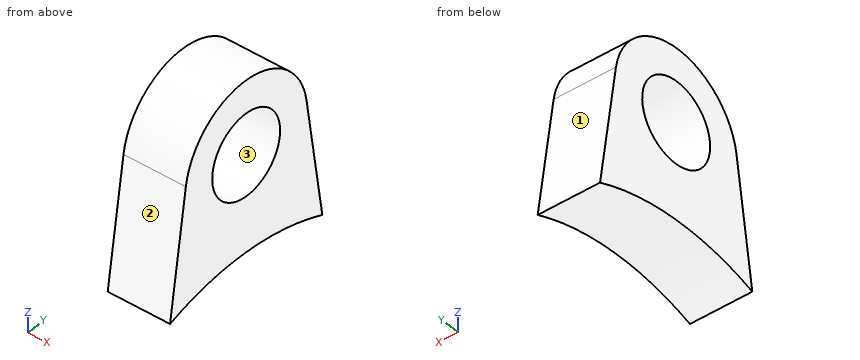
```python
from build123d import *

# Parameters (mm, degrees)
SZKIC19_R                   = 3.2
DODANIE_WYCI_GNI_CIE4_DEPTH = 5


with BuildPart() as part:
    # Szkic19 → Dodanie-wyciągnięcie4 (new body)
    with BuildSketch(Plane(origin=(91.785447504, 0, 0), x_dir=(0, 0, -1), z_dir=(1, 0, 0))):
        with BuildLine():
            ThreePointArc((-28.445954588, 5.671654954), (-33.249878941, -0.037311688), (-28.372269859, -5.683453641))
            Line((-28.372269859, -5.683453641), (-18.66960621, -7.172573037))
            ThreePointArc((-18.66960621, -7.172573037), (-20, 0), (-18.66960621, 7.172573037))
            Line((-18.66960621, 7.172573037), (-28.445954588, 5.671654954))
        make_face()
        with Locations((-27.5, 0)):
            Circle(SZKIC19_R, mode=Mode.SUBTRACT)
    extrude(amount=-DODANIE_WYCI_GNI_CIE4_DEPTH)


solid = part.part
```
Geometry check sheet. Reference: the model listing, model coordinates, mm. Face numbers are marked on the shaded views. Give positions to 0.01 mm unless a question says otherwise; leave off trailing zeros. Loops run counter-clockwise (first coordinate to the right, second up) from the corner with the lowest first, then second, coordinate; pieces in that order, holes last. Notation, with made-up numbers: M 10,37.5 L 22,37.5 A18 cw 22,63.5 Z; hole C -25,-13.75 d7. An arc over 180 degrees is marked long. Write item = value, one per line.
(1) Gauge pin test, flat ends, axial feed: pin 1 Ø1 at (x, z) = (90.5, 25) entering from +Y; pin 2 Ø1 at (x, z) = (91, 23) entering from +Y; pin 3 Ø4 at (y, z) = (0, 27.5) entering from -X; pin 4 Ø2 at (x, y) = (88, 5.5) entering from -Z. Record the tip position at first contact, or that the pin passes through.
Answer below:
pin_1 = 6.28
pin_2 = 6.58
pin_3 = through
pin_4 = 18.91
(2) Sectioned sample at A-A, the plane x = 88.5. Record the cut outline in (y, z).
Answer below:
outline = M -7.17,18.67 A20 cw 7.17,18.67 L 5.67,28.45 A5.75 ccw -5.68,28.37 Z; hole C 0,27.5 d6.4
(3) Material ranges on line 1 (Y direction, x = 90.15, z = 27.5); line 2 (Y direction, x = 90.1, z = 26); line 3 (Z direction, x = 90.5, y = -1.5), recorded low to high. Write a range as [from, to].
Answer below:
line_1 = [-5.82, -3.2], [3.2, 5.82]
line_2 = [-6.05, -2.83], [2.83, 6.05]
line_3 = [19.94, 24.67], [30.33, 33.05]
(4) Sectioned sample at C-C, the plane z = 24.75. Record the cut outline in (x, y).
Answer below:
outline = M 86.79,-6.24 L 91.79,-6.24 L 91.79,-1.64 L 86.79,-1.64 Z; M 86.79,1.64 L 91.79,1.64 L 91.79,6.24 L 86.79,6.24 Z
(5) Sectioned sample at B-B, the plane y = 0. Record the cut outline in (x, z).
Answer below:
outline = M 86.79,20 L 91.79,20 L 91.79,24.3 L 86.79,24.3 Z; M 86.79,30.7 L 91.79,30.7 L 91.79,33.25 L 86.79,33.25 Z
(6) Release check for a two-part mould opening along Y. For the marked faces 1, 2 and 3 record: released by +Y, released by -Y, zero draft, split by the parting line, or undercut.
Answer below:
face_1 = released by +Y
face_2 = released by -Y
face_3 = undercut
(7) Sectioned sample at D-D, the plane z = 32. Record the cut outline in (x, y).
Answer below:
outline = M 86.79,-3.58 L 91.79,-3.58 L 91.79,3.58 L 86.79,3.58 Z
